Autodesk Fusion 360 part; units mm, degrees
sketch "草图1" plane through (0, 0, 0) normal (0, 0, 1) x (1, 0, 0)
  line L0 (0, 100) -> (0, -123.0461) construction
  line L1 (-180, 0) -> (103.1908, 0) construction
  arc A0 (14.5237, -26.25) -> (-14.5237, -26.25) centre (0, -40) ccw
  line L2 (-4, 29.7321) -> (-4, 15)
  line L3 (4, 15) -> (4, 29.7321)
  arc A1 (-4, 15) -> (0, 11) centre (0, 15) ccw
  arc A2 (0, 11) -> (4, 15) centre (0, 15) ccw
  line L4 (-14.9904, -4.0359) -> (-27.7488, -11.402)
  line L5 (-23.7488, -18.3302) -> (-10.9904, -10.9641)
  arc A3 (-10.9904, -10.9641) -> (-9.5263, -5.5) centre (-12.9904, -7.5) ccw
  arc A4 (-9.5263, -5.5) -> (-14.9904, -4.0359) centre (-12.9904, -7.5) ccw
  arc A5 (15.4713, 25.7029) -> (29.995, 0.5471) centre (34.641, 20) ccw
  line L6 (10.9904, -10.9641) -> (23.7488, -18.3302)
  line L7 (27.7488, -11.402) -> (14.9904, -4.0359)
  arc A6 (14.9904, -4.0359) -> (9.5263, -5.5) centre (12.9904, -7.5) ccw
  arc A7 (9.5263, -5.5) -> (10.9904, -10.9641) centre (12.9904, -7.5) ccw
  arc A8 (-29.995, 0.5471) -> (-15.4713, 25.7029) centre (-34.641, 20) ccw
  arc A9 (15.4713, 25.7029) -> (4, 29.7321) centre (0, 0) ccw
  arc A10 (-4, 29.7321) -> (-15.4713, 25.7029) centre (0, 0) ccw
  arc A11 (27.7488, -11.402) -> (29.995, 0.5471) centre (0, 0) ccw
  arc A12 (14.5237, -26.25) -> (23.7488, -18.3302) centre (0, 0) ccw
  arc A13 (-29.995, 0.5471) -> (-27.7488, -11.402) centre (0, 0) ccw
  arc A14 (-23.7488, -18.3302) -> (-14.5237, -26.25) centre (0, 0) ccw
  circle A15 centre (0, 0) radius 7.5
  circle A16 centre (0, 0) radius 10
  point P0 (-4, 11)
  point P1 (4, 11)
  dimension "d2" = 20
  dimension "d3" = 40
  dimension "d4" = 60
  dimension "d6" = 8
  dimension "d8" = 4
  dimension "d10" = 360
  dimension "d11" = 15
  dimension "d12" = 20
extrude "拉伸1" add sketch "草图1" along normal blind 6 contours A0 L2 L3 A1 A2 L4 L5 A3 A4 A5 L6 L7 A6 A7 A8 A9 A10 A11 A12 A13 A14
sketch "草图2" plane through (0, 0, 0) normal (0, 0, 1) x (1, 0, 0)
  circle A0 centre (0, 0) radius 10
ref_plane "工作平面1" through (0, 0, 9) normal (0, 0, 1) x (1, 0, 0)
sketch "草图3" plane through (0, 0, 9) normal (0, 0, 1) x (1, 0, 0)
  circle A0 centre (0, 0) radius 7.5
  circle A1 centre (0, 0) radius 6
  dimension "d16" = 15
  dimension "d17" = 12
extrude "拉伸2" add sketch "草图2" along normal blind 6
sketch "草图4" plane through (0, 0, 6) normal (0, 0, 1) x (-1, 0, 0)
  line L0 (10.9904, 10.9641) -> (23.7488, 18.3302)
  arc A0 (23.7488, 18.3302) -> (14.5237, 26.25) centre (0, 0) ccw
  arc A1 (-14.5237, 26.25) -> (14.5237, 26.25) centre (0, 40) ccw
  arc A2 (-14.5237, 26.25) -> (-23.7488, 18.3302) centre (0, 0) ccw
  line L1 (-23.7488, 18.3302) -> (-10.9904, 10.9641)
  arc A3 (-14.9904, 4.0359) -> (-10.9904, 10.9641) centre (-12.9904, 7.5) ccw
  line L2 (-14.9904, 4.0359) -> (-27.7488, 11.402)
  arc A4 (-27.7488, 11.402) -> (-29.995, -0.5471) centre (0, 0) ccw
  arc A5 (-15.4713, -25.7029) -> (-29.995, -0.5471) centre (-34.641, -20) ccw
  arc A6 (-15.4713, -25.7029) -> (-4, -29.7321) centre (0, 0) ccw
  line L3 (-4, -29.7321) -> (-4, -15)
  arc A7 (4, -15) -> (-4, -15) centre (0, -15) ccw
  line L4 (4, -15) -> (4, -29.7321)
  arc A8 (4, -29.7321) -> (15.4713, -25.7029) centre (0, 0) ccw
  arc A9 (29.995, -0.5471) -> (15.4713, -25.7029) centre (34.641, -20) ccw
  arc A10 (29.995, -0.5471) -> (27.7488, 11.402) centre (0, 0) ccw
  line L5 (27.7488, 11.402) -> (14.9904, 4.0359)
  arc A11 (10.9904, 10.9641) -> (14.9904, 4.0359) centre (12.9904, 7.5) ccw
  circle A12 centre (0, 0) radius 10
loft "放样1" add profiles "草图4", "草图3" section 1 contours A12 section 2
extrude "拉伸3" cut sketch "草图3" against normal blind 21 contours A1
mirror "镜像1" about plane through (0, 0, 0) normal (0, 0, 1) of bodies 1 merged
Source: CAD feature listing. Evaluate the final solid. Frame: model axes, mm. A direction names the side the tool comes from. Round coordinates to 2 decimals unless told otherwise and drop trailing zeros. Loops run counter-clockwise (first coordinate to the right, second up) from the corner with the lowest first, then second, coordinate; pieces in that order, holes last. Notation, with made-up numbers: (-28, -6) - (21, -6) arc R20 ccw to (21, 5) - close; hole circle Ø4 at (39.25, 75). An arc over 180 degrees is marked (long way). Use CSV: the item, a comma, the result in double quotes.
Q1. Section query D-D, the plane x = 23. Output: boundary loops of the cut face in (y, z).
Reported:
outline,"(-19.26, -6) - (-17.9, -6) - (-17.9, 6) - (-19.26, 6) - close; (-8.66, -6) - (3.74, -6) - (3.74, 6) - (-8.66, 6) - close"
Q2. Pin query (flat end, axial travel): pin 1 Ø3 at (y, z) = (21.5, 6.5) entering from +X; pin 2 Ø3 at (x, z) = (9, -7) entering from +Y; pin 3 Ø3.5 at (y, z) = (26, -1.5) entering from -X. Return the tip coordinate at first contact, or that it passes through.
Reported:
pin 1,"x = 14.85"
pin 2,"y = 28.95"
pin 3,"x = -15.47"
Q3. Section query C-C, the plane y = -22. Output: boundary loops of the cut face in (x, z).
Reported:
outline,"(-20.4, -6) - (-8.72, -6) - (-8.72, 6) - (-20.4, 6) - close; (8.72, -6) - (20.4, -6) - (20.4, 6) - (8.72, 6) - close"
Q4. Reachability of faces 5 (the cylindrical face through (-19.5, -22.8, -0.1)), 6 (the flat face through (-6.2, 8.4, -6)), 7 (the flat face through (-4, 22, 0)) from +Z, -Z, +X, -X, +Y, -Y: full face, straight path, thin tool, end or side. Return the list, or none.
Reported:
face 5,"+Z, -Z, -X, -Y"
face 6,"-Z"
face 7,"+Z, -Z, +Y"
Q5. Section query A-A, the plane z = 4.5. Output: boundary loops of the cut face in (x, y) (3 decimals), then the cut area to 3 significant figures.
Reported:
outline,"(-29.995, 0.547) arc R30 ccw to (-27.749, -11.402) - (-14.99, -4.036) arc R4 cw to (-10.99, -10.964) - (-23.749, -18.33) arc R30 ccw to (-14.524, -26.25) arc R20 cw to (14.524, -26.25) arc R30 ccw to (23.749, -18.33) - (10.99, -10.964) arc R4 cw to (14.99, -4.036) - (27.749, -11.402) arc R30 ccw to (29.995, 0.547) arc R20 cw to (15.471, 25.703) arc R30 ccw to (4, 29.732) - (4, 15) arc R4 cw to (-4, 15) - (-4, 29.732) arc R30 ccw to (-15.471, 25.703) arc R20 cw to start; hole circle Ø12 at (0, 0)"
area,"1,680 mm^2"
Q6. Mould query, pull axis Y, two halves, no side actions, for faces 1 (the flat face through (-21.28, -7.667, -0.084)), 2 (the flat face through (21.46, -7.77, -0.08)), 3 (the cylindrical face through (19.607, -22.706, -0.084)), 4 (the flat face through (-2, 6, -9)). Classes: pulls with the +Y half, pulls with the -Y half, needs draft (parallel to the pull), parting line crosses it, or undercut.
Reported:
face 1,"undercut"
face 2,"undercut"
face 3,"pulls with the -Y half"
face 4,"needs draft"
Q7. Section query B-B, the plane x = 0. Output: boundary loops of the cut face in (y, z), then the cut area to 3 significant figures.
Reported:
outline,"(-20, -6) - (-10, -6) - (-7.5, -9) - (-6, -9) - (-6, 9) - (-7.5, 9) - (-10, 6) - (-20, 6) - close; (6, -9) - (7.5, -9) - (10, -6) - (11, -6) - (11, 6) - (10, 6) - (7.5, 9) - (6, 9) - close"
area,"261 mm^2"
Q8. Ray query, line 1 along Y through (x, z) = (0, -4.5); line 2 along Z through (x, y) = (-9, 19.5); line 3 along X through (y, z) = (-23, -3.25). Return the intervals inside material, ascending.
Reported:
line 1,"-20 to -6, 6 to 11"
line 2,"-6 to 6"
line 3,"-19.26 to -10.54, 10.54 to 19.26"
